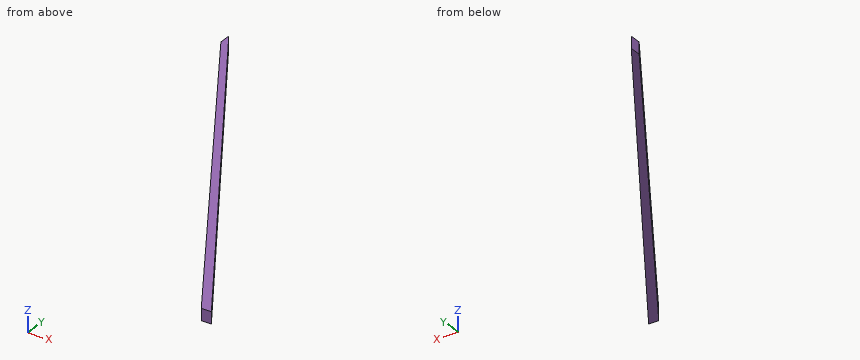
```python
from build123d import *

# Parameters (mm, degrees)
BOSS_EXTRUDE1_DEPTH = 25.4
CUT_EXTRUDE2_DEPTH  = 127
CUT_EXTRUDE3_DEPTH  = 127


with BuildPart() as part:
    # Sketch1 → Boss-Extrude1 (new body)
    with BuildSketch(Plane.XY):
        Polygon((0, 830.58), (515.62, 0), (494.040159482, -13.396659404), (0, 782.421725573), align=None)
    extrude(amount=-BOSS_EXTRUDE1_DEPTH)

    # Sketch2 → Cut-Extrude2 (cut)
    with BuildSketch(Plane.XY):
        Polygon((515.62, 0), (485.723578873, 0), (494.040159482, -13.396659404), align=None)
    extrude(amount=-CUT_EXTRUDE2_DEPTH, mode=Mode.SUBTRACT)

    # Sketch4 → Cut-Extrude3 (cut)
    with BuildSketch(Plane(origin=(0, 0, -25.4), x_dir=(-1, 0, 0), z_dir=(0, 0, -1))):
        Polygon((0, 805.281725573), (-493.978617069, 0), (-485.723578873, 0), (0, 782.421725573), align=None)
    extrude(amount=-CUT_EXTRUDE3_DEPTH, mode=Mode.SUBTRACT)


solid = part.part
```
Geometry check sheet. Reference: the model listing, model coordinates, mm. Coordinates: 2 decimals unless noted, no trailing zeros. Write each loop counter-clockwise with the first axis right and the second up, starting at its lowest first coordinate (ties: lowest second). Pieces come first, ordered by that corner, then holes. Notation, with made-up numbers: M 83,15.5 L 140,15.5 A23 cw 140,32.5 Z; hole C 41,70.25 d2. An arc over 180 degrees is marked long. One line per item, written item: value. Start each with the question number.
(1) Sectioned sample at A-A, the plane z = -12.75. Enter the section's corners in (x, y).
(2) Scan lines: line 1 along Y through (x, z) = (145, -21.5); line 2 along Y through (x, z) = (212, -11.5); line 3 along X through (y, z) = (288, -8.5). Record each from-to range of solid material in increasing order. Write a range as [from, to].
(3) Sectioned sample at B-B, the plane y = 514. Enter the section's corners in (x, z).
(4) Depth check by flat-ended pin: pin 1 (1 mm diameter, centred on x = 237, z = -22, fed in from +Y); pin 2 (3 mm diameter, centred on y = 156, z = -11, fed in from +X); pin 3 (6 mm diameter, centred on x = 165, z = -11, fed in from +Y). Enter the tip coordinate at first touch or a pass-through.
Filled sheet:
1. outline: M 0,805.28 L 493.98,0 L 515.62,0 L 0,830.58 Z
2. line 1: [568.9, 597.01]
2. line 2: [459.68, 489.08]
2. line 3: [317.31, 336.83]
3. outline: M 178.68,-25.4 L 196.53,-25.4 L 196.53,0 L 178.68,0 Z
4. pin 1: y = 449.62
4. pin 2: x = 419.71
4. pin 3: y = 569.62
